```python
from build123d import *

# Parameters (mm, degrees)
BOSS_EXTRUDE2_DEPTH = 0.6


with BuildPart() as part:
    # Sketch2 → Boss-Extrude2 (new body)
    with BuildSketch(Plane.XY):
        with BuildLine():
            ThreePointArc((2.074223627, -15.871495922), (1.151683238, -16.599881603), (0, -16.834939442))
            ThreePointArc((0, -16.834939442), (-1.151683238, -16.599881603), (-2.074223627, -15.871495922))
            ThreePointArc((-2.074223627, -15.871495922), (-8.410066736, -6.972099792), (-13.820679581, 2.518286292))
            ThreePointArc((-13.820679581, 2.518286292), (-13.991707448, 10.221670001), (-8.106427403, 15.195084311))
            ThreePointArc((-8.106427403, 15.195084311), (-4.08641149, 15.955883205), (0, 16.157338))
            ThreePointArc((0, 16.157338), (4.08641149, 15.955883205), (8.106427403, 15.195084311))
            ThreePointArc((8.106427403, 15.195084311), (13.991707448, 10.221670001), (13.820679581, 2.518286292))
            ThreePointArc((13.820679581, 2.518286292), (8.410066736, -6.972099792), (2.074223627, -15.871495922))
        make_face()
    extrude(amount=BOSS_EXTRUDE2_DEPTH)


solid = part.part
```
For this review, take the finished solid that the model builds, in its own axes (mm). Coordinates: 2 decimals unless noted, no trailing zeros. Write each loop counter-clockwise with the first axis right and the second up, starting at its lowest first coordinate (ties: lowest second). Pieces come first, ordered by that corner, then holes.
(1) Add section A-A on z = 0.2. Give the boundary of the cut face in (x, y), then the cut area to 3 significant figures.
(2) Wall thickness on probe 1 along X at (y, z) = (-3, 0.3); probe 2 along X at (y, z) = (13.5, 0.4); probe 3 along Y at (x, z) = (12, 0.55): over which ranges is each line inside the solid? List them lowest first.
(3) Add section C-C on x = -8.5. Give the boundary of the cut face in (y, z).
(4) Add section B-B on y = -2.5. Give the boundary of the cut face in (x, z), then the cut area to 3 significant figures.
Answer sheet:
1. outline: (-13.82, 2.52) arc R108.7 ccw to (-2.07, -15.87) arc R2.54 ccw to (0, -16.83) arc R2.54 ccw to (2.07, -15.87) arc R108.7 ccw to (13.82, 2.52) arc R8.94 ccw to (8.11, 15.2) arc R29.72 ccw to (0, 16.16) arc R29.72 ccw to (-8.11, 15.2) arc R8.94 ccw to start
1. area: 664 mm2
2. probe 1: x = -10.83 to 10.83
2. probe 2: x = -11.46 to 11.46
2. probe 3: y = -0.93 to 13.03
3. outline: (-6.83, 0) - (15.08, 0) - (15.08, 0.6) - (-6.83, 0.6) - close
4. outline: (-11.12, 0) - (11.12, 0) - (11.12, 0.6) - (-11.12, 0.6) - close
4. area: 13.3 mm2
